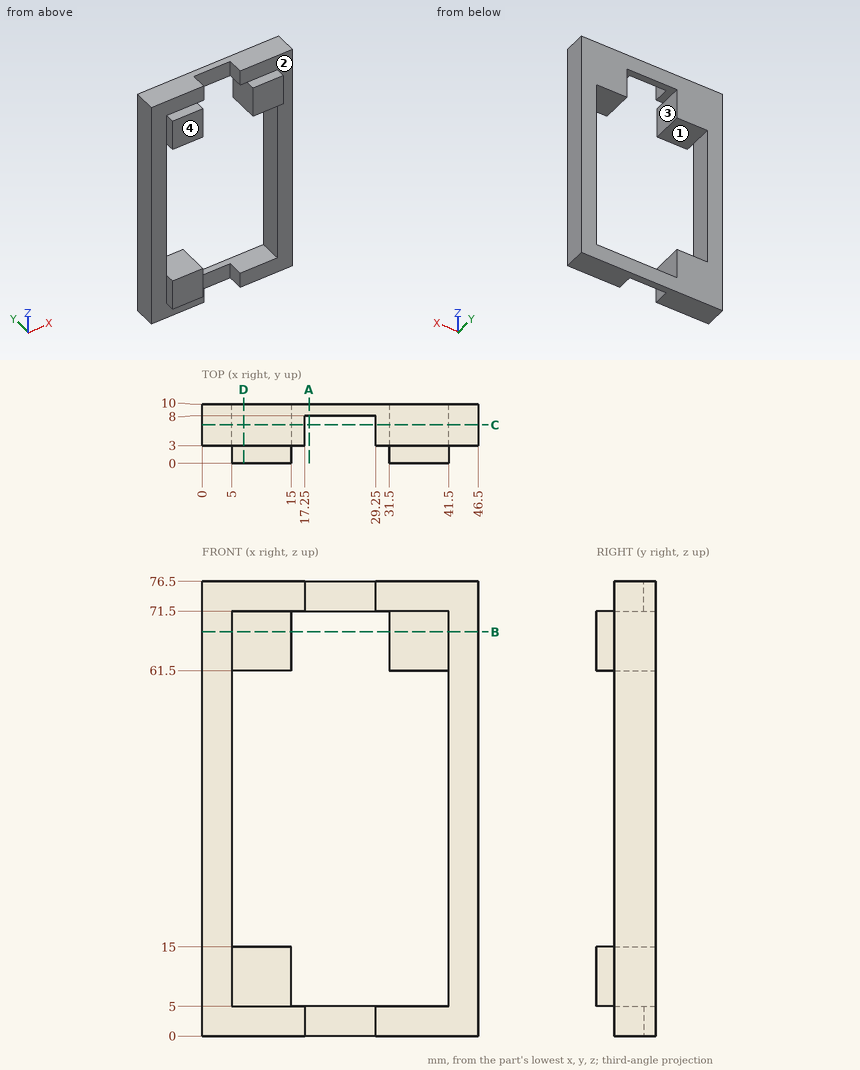
Design review of the part shown in the three views and the two pictorial views. Dimensions are in mm from the part's minimum x, y and z. A direction names the side the tool comes from. Give positions to 0.01 mm unless a question says otherwise; leave off trailing zeros. Write each loop counter-clockwise with the first axis right and the second up, starting at its lowest first coordinate (ties: lowest second). Pieces come first, ordered by that corner, then holes.
(1) Wall thickness on line 1 along Z through (x, y) = (32, 4); line 2 along X through (y, z) = (6, 48); line 3 along Z through (x, y) = (25, 9.25): over which ranges is each line inside the solid? List them lowest first.
Checked values:
line 1: z = 0 to 5, 61.5 to 76.5
line 2: x = 0 to 5, 41.5 to 46.5
line 3: z = 0 to 5, 71.5 to 76.5
(2) Clearance check with flat-ended pins moving along their axes: pin 1 Ø3.5 at (x, y) = (24, 5.5) entering from +Z; pin 2 Ø1.5 at (x, y) = (11.5, 2) entering from +Z; pin 3 Ø4 at (x, z) = (40.5, 34) entering from -Y; pin 4 Ø0.9 at (y, z) = (1.5, 8) entering from -X. State where each tip first meets the part, or that it passes through.
Checked values:
pin 1: passes through
pin 2: stops at z = 71.5
pin 3: stops at y = 3
pin 4: stops at x = 5
(3) Tool access review of the marked faces 3 and 4: name each direction out of +Z, -Z, +X, -X, +Y, -Y from which nothing blocks a thin tool from reaching the whole face with its end or side.
Checked values:
face 3: +Y, -Y
face 4: +Z, -Z, +X, -X, -Y
(4) Add section D-D (x = 7). Give the boundary of the cut face in (y, z), and give its area (3 significant figures).
Checked values:
outline: (0, 5) - (3, 5) - (3, 0) - (10, 0) - (10, 15) - (0, 15) - close; (0, 61.5) - (10, 61.5) - (10, 76.5) - (3, 76.5) - (3, 71.5) - (0, 71.5) - close
area: 270 mm2
(5) Add section C-C (y = 6.5). Give the boundary of the cut face in (x, z).
Checked values:
outline: (0, 0) - (17.25, 0) - (17.25, 5) - (15, 5) - (15, 15) - (5, 15) - (5, 61.5) - (15, 61.5) - (15, 71.5) - (17.25, 71.5) - (17.25, 76.5) - (0, 76.5) - close; (29.25, 0) - (46.5, 0) - (46.5, 76.5) - (29.25, 76.5) - (29.25, 71.5) - (31.5, 71.5) - (31.5, 61.5) - (41.5, 61.5) - (41.5, 5) - (29.25, 5) - close
(6) Add section A-A (x = 18). Give the boundary of the cut face in (y, z).
Checked values:
outline: (8, 0) - (10, 0) - (10, 5) - (8, 5) - close; (8, 71.5) - (10, 71.5) - (10, 76.5) - (8, 76.5) - close
(7) Mouldability with a two-part tool opening along X and no side actions: class the marked faces 1 and 2 as +X half, -X half, draft (parallel to the pull), parting line (faces both ways), or undercut.
Checked values:
face 1: undercut
face 2: draft
(8) Add section B-B (z = 68). Give the boundary of the cut face in (x, y), and give its area (3 significant figures).
Checked values:
outline: (0, 3) - (5, 3) - (5, 0) - (15, 0) - (15, 10) - (0, 10) - close; (31.5, 0) - (41.5, 0) - (41.5, 3) - (46.5, 3) - (46.5, 10) - (31.5, 10) - close
area: 270 mm2
